```python
from build123d import *

# Parameters (mm, degrees)
F1_W     = 35
F1_H     = 35
F2_DEPTH = 10
F3_R     = 3
F4_W     = 30
F4_H     = 20
F4_R     = 1
F4_W_2   = 20
F4_H_2   = 30
F5_DEPTH = 5
F6_R     = 3
F8_D     = 3.3


with BuildPart() as f2:
    # F1 (on offset) → F2 (new body)
    with BuildSketch(Plane.XY.offset(9)):
        Rectangle(F1_W, F1_H)
    extrude(amount=F2_DEPTH)

    # F3
    f3_edges = [f2.edges().sort_by_distance(p)[0] for p in [
        (-17.5, -17.5, 14),
        (17.5, -17.5, 14),
        (17.5, 17.5, 14),
        (-17.5, 17.5, 14),
    ]]
    fillet(f3_edges, radius=F3_R)

    # F4 (on offset) → F5 (join)
    with BuildSketch(Plane.XY.offset(9)):
        with Locations((32.5, 0)):
            Rectangle(F4_W, F4_H)
        with Locations((30, 0)):
            Circle(F4_R, mode=Mode.SUBTRACT)
        with Locations((40, 0)):
            Circle(F4_R, mode=Mode.SUBTRACT)
        with Locations((-32.5, 0)):
            Rectangle(F4_W, F4_H)
        with Locations((-40, 0)):
            Circle(F4_R, mode=Mode.SUBTRACT)
        with Locations((-30, 0)):
            Circle(F4_R, mode=Mode.SUBTRACT)
        with Locations((0, -32.5)):
            Rectangle(F4_W_2, F4_H_2)
        with Locations((0, -40)):
            Circle(F4_R, mode=Mode.SUBTRACT)
        with Locations((0, -30)):
            Circle(F4_R, mode=Mode.SUBTRACT)
        with Locations((0, 32.5)):
            Rectangle(F4_W_2, F4_H_2)
        with Locations((0, 30)):
            Circle(F4_R, mode=Mode.SUBTRACT)
        with Locations((0, 40)):
            Circle(F4_R, mode=Mode.SUBTRACT)
    extrude(amount=F5_DEPTH)

    # F6
    f6_edges = [f2.edges().sort_by_distance(p)[0] for p in [
        (-47.5, 10, 11.5),
        (-47.5, -10, 11.5),
        (-10, -47.5, 11.5),
        (10, -47.5, 11.5),
        (47.5, -10, 11.5),
        (47.5, 10, 11.5),
        (10, 47.5, 11.5),
        (-10, 47.5, 11.5),
    ]]
    fillet(f6_edges, radius=F6_R)

    # F8 (through all)
    with Locations(Plane.XY.offset(19)):
        with Locations((-12, 12), (12, 12), (12, -12), (-12, -12)):
            Hole(F8_D / 2)


solid = f2.part
```
Work out the finished part from the listing and answer in its coordinate system (mm). A direction names the side the tool comes from. Round coordinates to 2 decimals unless told otherwise and drop trailing zeros. Write each loop counter-clockwise with the first axis right and the second up, starting at its lowest first coordinate (ties: lowest second). Pieces come first, ordered by that corner, then holes.
1) Consider probe 1 along Y at (x, z) = (12, 11); probe 2 along Y at (x, z) = (0, 11.7); probe 3 along X at (y, z) = (0.5, 11). Determine where each line is inside the solid, lowest interval first.
2) Determine the mould class of faces 4 (the face through (-9.14, 46.6, 11.54)), 5 (the face through (0, 33, 14)), 6 (the face through (-13.524, -12.632, 13.93)) for opening direction X: pulls with the +X half, pulls with the -X half, needs draft (parallel to the pull), parting line crosses it, or undercut.
3) Which of the six approach directions +Z, -Z, +X, -X, +Y, -Y give full straight-line access (tool end or side, diameter ignored) to faces 1 (the face through (10, 31, 11)), 2 (the face through (32, 0, 14)), 3 (the face through (0, -32, 14))?
4) Flat-ended cylindrical pins translate along their axes: P1, Ø10, axis at x = -4.5, y = -31.5, coming from the +Z side; P2, Ø4, axis at y = -13.5, z = 17, coming from the +X side; P3, Ø1.5, axis at x = -8.5, z = 18, coming from the -Y side. Find the tip coordinate at first contact, or state that the pin passes through.
5) A cutting plane is placed at C-C on x = -37. Determine the outline of the cut face in (y, z).
6) A cutting plane is placed at B-B on z = 12.25. Give the number of separate pieces and of enclosed holes in the cut face, and give its area (3 significant figures).
7) A cutting plane is placed at A-A on y = 12. Determine the outline of the cut face in (x, z), and give its area (3 significant figures).
Entries:
1. probe 1: y = -17.5 to -13.65, -10.35 to 10.35, 13.65 to 17.5
1. probe 2: y = -47.5 to -41, -39 to -31, -29 to 29, 31 to 39, 41 to 47.5
1. probe 3: x = -47.5 to -40.87, -39.13 to -30.87, -29.13 to 29.13, 30.87 to 39.13, 40.87 to 47.5
2. face 4: pulls with the -X half
2. face 5: needs draft
2. face 6: undercut
3. face 1: +Z, -Z, +X, +Y
3. face 2: +Z, +X, +Y, -Y
3. face 3: +Z, +X, -X, -Y
4. P1: stops at z = 14
4. P2: stops at x = 17.5
4. P3: stops at y = -17.5
5. outline: (-10, 9) - (10, 9) - (10, 14) - (-10, 14) - close
6. separate pieces: 1
6. enclosed holes: 12
6. area: 3,540 mm2
7. outline: (-17.5, 9) - (-13.65, 9) - (-13.65, 19) - (-17.5, 19) - close; (-10.35, 9) - (10.35, 9) - (10.35, 19) - (-10.35, 19) - close; (13.65, 9) - (17.5, 9) - (17.5, 19) - (13.65, 19) - close
7. area: 284 mm2
